Source: CAD feature listing. Evaluate the final solid. Frame: model axes, mm. Face numbers are marked on the shaded views. A direction names the side the tool comes from. Give positions to 0.01 mm unless a question says otherwise; leave off trailing zeros. Order: outer loops, then holes, each group sorted by start corner. A loop starts at its lowest first (then second) coordinate and runs counter-clockwise, first axis right, second up.
1) Section A-A, the plane x = 4. Return loops of the section in (y, z), plus the area to 3 significant figures.
2) Access query for the marked faces 1, 2, 3 and 4. Directions: +Z, -Z, +X, -X, +Y, -Y. A direction counts if a zero-diameter tool reaches every point of the face in a straight line with its end or side. Return the directions, or none.
3) Material intervals for line 1 (Y direction, x = 5.5, z = -0.5); line 2 (X direction, y = 24, z = 5.75); line 3 (X direction, y = 31.5, z = 5.75), sorted ascending.
4) Section D-D, the plane y = 25.5. Return loops of the section in (x, z), plus the area to 3 significant figures.
5) Section B-B, the plane z = 4.5. Return loops of the section in (x, y).
6) Section C-C, the plane x = 11.5. Return loops of the section in (y, z), plus the area to 3 significant figures.
7) Draft query along Y for the marked faces 5, 6 and 7. Return one class per face: released by +Y, released by -Y, zero draft, split by the parting line, or undercut.
8) First-contact query: P1, Ø4, axis at y = 8.5, z = 3, coming from the -X side; P2, Ø4, axis at y = 35.5, z = 1.5, coming from the +X side; P3, Ø8, axis at y = 33.5, z = 5, coming from the +X side; P4, Ø1, axis at x = 10, y = 26, coming from the -Z side. Flat tips, straight axial feed; report the tip coordinate or a pass-through.
```python
from build123d import *

# Parameters (mm, degrees)
ESBO_O1_W                = 3
ESBO_O1_H                = 50.4
RESSALTO_EXTRUS_O1_DEPTH = 7
FILETE1_R                = 2
RESSALTO_EXTRUS_O2_DEPTH = 14
FILETE2_R                = 1


with BuildPart() as part:
    # Esboço1 → Ressalto-extrusão1 (new body, symmetric)
    with BuildSketch(Plane.XY):
        with Locations((0, 25.2)):
            Rectangle(ESBO_O1_W, ESBO_O1_H)
        Polygon((-7.5, 0), (-1.5, 0), (-1.5, 4), (-7.5, 2), align=None)
        Polygon((1.5, 4), (1.5, 0), (7.5, 0), (7.5, 2), align=None)
    extrude(amount=RESSALTO_EXTRUS_O1_DEPTH, both=True)

    # Filete1
    filete1_edges = [part.edges().sort_by_distance(p)[0] for p in [
        (-7.5, 1, -7),
        (7.5, 1, -7),
        (7.5, 1, 7),
        (-7.5, 1, 7),
    ]]
    fillet(filete1_edges, radius=FILETE1_R)

    # Esboço3 → Ressalto-extrusão2 (add)
    with BuildSketch(Plane(origin=(1.5, 0, 0), x_dir=(0, 0, -1), z_dir=(1, 0, 0))):
        with BuildLine():
            Line((-7, 32.573762079), (-7, 30.043842411))
            ThreePointArc((-7, 30.043842411), (0, 27.9), (7, 30.043842411))
            Line((7, 30.043842411), (7, 32.573762079))
            ThreePointArc((7, 32.573762079), (0, 29.9), (-7, 32.573762079))
        make_face()
    extrude(amount=RESSALTO_EXTRUS_O2_DEPTH)

    # Filete2
    filete2_edges = [part.edges().sort_by_distance(p)[0] for p in [
        (15.5, 31.308802245, 7),
        (15.5, 31.308802245, -7),
    ]]
    fillet(filete2_edges, radius=FILETE2_R)


solid = part.part
```
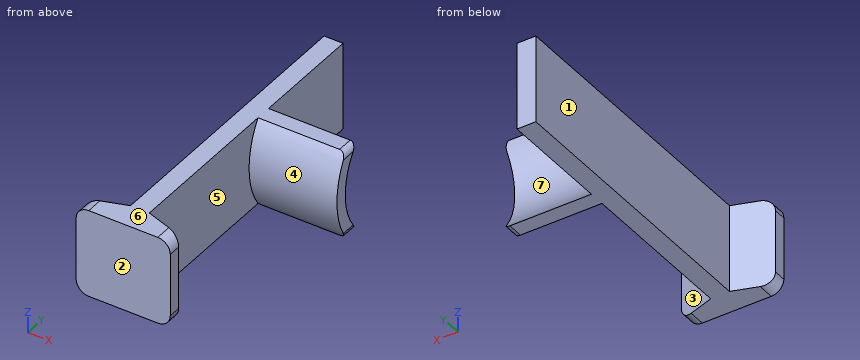
From the geometry:
1. outline: (0, -7) - (3.17, -7) - (3.17, 7) - (0, 7) - close; (30.04, -7) - (32.57, -7) arc R10.5 cw to (32.57, 7) - (30.04, 7) arc R12.5 ccw to start
1. area: 74.5 mm2
2. face 1: +Z, -Z, -X, +Y
2. face 2: +Z, -Z, +X, -X, -Y
2. face 3: +Z, -Z, +X
2. face 4: +X
3. line 1: y = 0 to 2.67, 27.91 to 29.91
3. line 2: x = -1.5 to 1.5
3. line 3: x = -1.5 to 15.5
4. outline: (-1.5, -7) - (1.5, -7) - (1.5, 7) - (-1.5, 7) - close
4. area: 42.0 mm2
5. outline: (-7.5, 0) - (7.5, 0) - (7.5, 2) - (1.5, 4) - (1.5, 28.74) - (15.5, 28.74) - (15.5, 30.91) - (1.5, 30.91) - (1.5, 50.4) - (-1.5, 50.4) - (-1.5, 4) - (-7.5, 2) - close
6. outline: (30.04, -7) - (32.57, -7) arc R10.5 cw to (32.57, 7) - (30.04, 7) arc R12.5 ccw to start
6. area: 30.1 mm2
7. face 5: undercut
7. face 6: zero draft
7. face 7: released by +Y
8. P1: stops at x = -1.5
8. P2: stops at x = 1.5
8. P3: stops at x = 15.5
8. P4: passes through
